```python
from build123d import *

# Parameters (mm, degrees)
FILLET1_R          = 1
CUT_EXTRUDE1_DEPTH = 3


with BuildPart() as part:
    # Sketch1 → Revolve2 (revolve)
    with BuildSketch(Plane.XY):
        Polygon((-124, 0), (-124, 10), (-54, 10), (-54, 15), (-30, 15), (-30, 20), (30, 20), (30, 15), (54, 15), (54, 10), (89, 10), (89, 0), align=None)
    revolve(axis=Axis((89, 0, 0), (-1, 0, 0)))

    # Fillet1
    fillet1_edges = [part.edges().sort_by_distance(p)[0] for p in [
        (30, -15, 0),
        (-30, -15, 0),
    ]]
    fillet(fillet1_edges, radius=FILLET1_R)

    # Sketch2 → Cut-Extrude1 (cut)
    with BuildSketch(Plane(origin=(0, 20, 0), x_dir=(1, 0, 0), z_dir=(0, 1, 0))):
        with BuildLine():
            Line((9, -6), (-9, -6))
            ThreePointArc((-9, -6), (-15, 0), (-9, 6))
            Line((-9, 6), (9, 6))
            ThreePointArc((9, 6), (15, 0), (9, -6))
        make_face()
    extrude(amount=-CUT_EXTRUDE1_DEPTH, mode=Mode.SUBTRACT)


solid = part.part
```
Geometry: final body of the model. Coordinates: model frame, mm. A direction names the side the tool comes from. Round coordinates to 2 decimals unless told otherwise and drop trailing zeros. Loops run counter-clockwise (first coordinate to the right, second up) from the corner with the lowest first, then second, coordinate; pieces in that order, holes last.
Item 1: Section A-A, the plane z = 0. Output: boundary loops of the cut face in (x, y).
Checked values:
outline: (-124, -10) - (-54, -10) - (-54, -15) - (-31, -15) arc R1 cw to (-30, -16) - (-30, -20) - (30, -20) - (30, -16) arc R1 cw to (31, -15) - (54, -15) - (54, -10) - (89, -10) - (89, 10) - (54, 10) - (54, 15) - (31, 15) arc R1 cw to (30, 16) - (30, 20) - (15, 20) - (15, 17) - (-15, 17) - (-15, 20) - (-30, 20) - (-30, 16) arc R1 cw to (-31, 15) - (-54, 15) - (-54, 10) - (-124, 10) - close
Item 2: Section D-D, the plane x = -4. Output: boundary loops of the cut face in (y, z).
Checked values:
outline: (17, -6) - (17, 6) - (19.08, 6) arc R20 ccw (long way) to (19.08, -6) - close
Item 3: Section C-C, the plane x = 18. Output: boundary loops of the cut face in (y, z).
Checked values:
outline: circle Ø40 at (0, 0)
Item 4: Contact query for flat-ended pins moving along their axis: P1, Ø3, axis at x = -6, y = -13, coming from the +Z side; P2, Ø1.5, axis at y = 11.5, z = 10, coming from the -X side; P3, Ø1.7, axis at x = -3.5, y = 17.5, coming from the -Z side. Output: stop coordinate, or through.
Checked values:
P1: stops at z = 16.36
P2: stops at x = -54
P3: stops at z = -11.08
Item 5: Mould query, pull axis Z, two halves, no side actions, for faces 6 (the cylindrical face through (15, 18, 0)), 7 (the flat face through (0, 17, 0)), 8 (the cylindrical face through (42.661, -14.985, -0.66)), 9 (the flat face through (54, 3, 10)). Classes: released by +Z, released by -Z, zero draft, split by the parting line, or undercut.
Checked values:
face 6: undercut
face 7: undercut
face 8: split by the parting line
face 9: zero draft
Item 6: Section B-B, the plane y = 0. Output: boundary loops of the cut face in (x, z).
Checked values:
outline: (-124, -10) - (-54, -10) - (-54, -15) - (-31, -15) arc R1 cw to (-30, -16) - (-30, -20) - (30, -20) - (30, -16) arc R1 cw to (31, -15) - (54, -15) - (54, -10) - (89, -10) - (89, 10) - (54, 10) - (54, 15) - (31, 15) arc R1 cw to (30, 16) - (30, 20) - (-30, 20) - (-30, 16) arc R1 cw to (-31, 15) - (-54, 15) - (-54, 10) - (-124, 10) - close
Item 7: Reachability of faces 1 (the flat face through (89, 0, 0)), 2 (the cylindrical face through (0.42, -4.336, 19.524)), 3 (the flat face through (-30, 8.98, -13.43)), 4 (the cylindrical face through (-15, 18, 0)), 5 (the flat face through (30, -8.98, -13.43)) from +Z, -Z, +X, -X, +Y, -Y: full face, straight path, thin tool, end or side. Return the list, or none.
Checked values:
face 1: +Z, -Z, +X, +Y, -Y
face 2: +X, -X
face 3: -X
face 4: +Y
face 5: +X
Item 8: Line query: L1, parallel to X at y = 6, z = 15; L2, parallel to Y at x = -48, z = -12; L3, parallel to X at y = 10, z = 10.5. Output: solid intervals per line, ascending.
Checked values:
L1: x = -30 to 30
L2: y = -9 to 9
L3: x = -54 to 54
